Design review of the part built by this model. Coordinates are the model's own, in mm. A direction names the side the tool comes from. Coordinates: 2 decimals unless noted, no trailing zeros. Loops run counter-clockwise (first coordinate to the right, second up) from the corner with the lowest first, then second, coordinate; pieces in that order, holes last. Notation, with made-up numbers: M 78,68.25 L 99,68.25 A18 ccw 99,84.25 Z; hole C 68,86 d2. An arc over 180 degrees is marked long. Answer as a JSON object with one key per item and string values. Group by question number.
1. Consider section C-C (x = 21). State the section outline as (y, z) points, then the cut area to 3 significant figures.
2. Consider section D-D (x = -24). State the section outline as (y, z) points, then the cut area to 3 significant figures.
3. Draft analysis for pull direction Y (two halves, no side actions). For faces 4 (the cylindrical face through (-26.68, 43.93, 5.15)), 5 (the flat face through (-1, 26, 10.16)), 6 (the cylindrical face through (-36.942, 49.272, 4.765)), state which applies: +Y half, -Y half, draft (parallel to the pull), parting line (faces both ways), or undercut.
4. To check wall thickness, follow probe 1 along X at (y, z) = (14, 2); probe 2 along X at (y, z) = (6, 5.5); probe 3 along Z at (x, y) = (-4.5, 31). State the ranges of each line that lie inside material, in increasing order.
5. Machinability: for faces 1 (the flat face through (-21.356, 24, 5)), 2 (the flat face through (-5.56, 16.14, 20.2)), 3 (the flat face through (1.766, 27.835, 21.408)), which of the approach directions +Z, -Z, +X, -X, +Y, -Y give a long, thin tool a straight path to every point of the face, cutting with its end or side? Answer none if there is none.
6. Consider section A-A (x = 29). State the section outline as (y, z) points.
7. Consider section B-B (y = 6.5). State the section outline as (x, z) points.
8. Insertion check: pin 1 (8 mm diameter, centred on x = -30.5, y = 24, fed in from +Z); pin 2 (5 mm diameter, centred on x = -1, y = 37.5, fed in from -Z); pin 3 (3 mm diameter, centred on x = 8.5, z = 20, fed in from -Y); pin 4 (5 mm diameter, centred on y = 39.5, z = 21, fed in from +X). Each pin has a flat end and moves straight along its axis. Give the tip position at first contact, or say it passes through.
from build123d import *

# Parameters (mm, degrees)
F0_W          = 76.2
F0_H          = 50.8
F1_DEPTH      = 10.16
F5_DEPTH      = 23.60986
F5_DEPTH_BACK = 6.00945
F7_DEPTH      = 25.4
F9_D          = 11.43
F9_DEPTH      = 127
F11_D         = 5.08
F11_DEPTH     = 127
F12_R         = 5.08
F13_SIZE      = 0.762
F14_R         = 2.54


with BuildPart() as f1:
    # F0 (on Top) → F1 (new body)
    with BuildSketch(Plane.XY):
        with Locations((-0.290839, 25.4)):
            Rectangle(F0_W, F0_H)
    extrude(amount=F1_DEPTH)

    # F4 (on face) → F5 (join, two sides)
    with BuildSketch(Plane(origin=(-3.34157, 3.876222, 14.060855), x_dir=(0.974746, 0.059349, 0.215288), z_dir=(-0.223318, 0.259049, 0.939693))) as f5_sk:
        Polygon((17.944019, 29.214139), (-2.262714, 12.845073), (2.102678, 7.456231), (22.309411, 23.825297), align=None)
    extrude(amount=F5_DEPTH)
    extrude(f5_sk.sketch, amount=-F5_DEPTH_BACK)

    # F6 (on face) → F7 (cut)
    with BuildSketch(Plane.XY.offset(10.16)):
        with BuildLine():
            ThreePointArc((-21.356091, 38.483839), (-26.801871, 43.92962), (-32.247651, 38.483839))
            Line((-32.247651, 38.483839), (-32.247651, 10.246455))
            ThreePointArc((-32.247651, 10.246455), (-26.801871, 4.800675), (-21.356091, 10.246455))
            Line((-21.356091, 10.246455), (-21.356091, 38.483839))
        make_face()
    extrude(amount=-F7_DEPTH, mode=Mode.SUBTRACT)

    # F9
    with Locations(Plane.XY.offset(10.16)):
        with Locations((28.977718, 9.68211)):
            Hole(F9_D / 2, depth=F9_DEPTH)

    # F11
    with Locations(Plane(origin=(-2.742742, 3.181581, -1.528896), x_dir=(0.789646, 0.553023, -0.265753), z_dir=(0.613563, -0.711733, 0.34202))):
        with Locations((8.980069, 37.900489)):
            Hole(F11_D / 2, depth=F11_DEPTH)

    # F12
    f12_edges = [f1.edges().sort_by_distance(p)[0] for p in [
        (37.809161, 0, 5.08),
        (37.809161, 50.8, 5.08),
        (-38.390839, 50.8, 5.08),
        (-38.390839, 0, 5.08),
    ]]
    fillet(f12_edges, radius=F12_R)

    # F13
    f13_edges = [f1.edges().sort_by_distance(p)[0] for p in [
        (-0.290839, 0, 10.16),
    ]]
    chamfer(f13_edges, length=F13_SIZE)

    # F14
    f14_edges = [f1.edges().sort_by_distance(p)[0] for p in [
        (-8.692086, 19.773218, 33.531991),
        (11.004337, 36.752892, 33.531991),
    ]]
    fillet(f14_edges, radius=F14_R)


solid = f1.part
Findings below:
{
 "1": {"outline": "M 0,0 L 50.8,0 L 50.8,9.4 L 50.04,10.16 L 0.76,10.16 L 0,9.4 Z", "area": "516 mm^2"},
 "2": {"outline": "M 0,0 L 5.58,0 L 5.58,10.16 L 0.76,10.16 L 0,9.4 Z; M 43.15,0 L 50.8,0 L 50.8,9.4 L 50.04,10.16 L 43.15,10.16 Z", "area": "134 mm^2"},
 "3": {"face 4": "undercut", "face 5": "draft", "face 6": "+Y half"},
 "4": {"probe 1": "x = -38.39 to -32.25, -21.36 to 25.23, 32.72 to 37.81", "probe 2": "x = -38.39 to -30.21, -23.39 to 24.61, 33.35 to 37.81", "probe 3": "z = 0 to 10.16"},
 "5": {"face 1": "+Z, -Z", "face 2": "+Z, -X, -Y", "face 3": "-X, +Y"},
 "6": {"outline": "M 0,0 L 3.97,0 L 3.97,10.16 L 0.76,10.16 L 0,9.4 Z; M 15.4,0 L 50.8,0 L 50.8,9.4 L 50.04,10.16 L 15.4,10.16 Z"},
 "7": {"outline": "M -38.39,0 L -30.75,0 L -30.75,10.16 L -37.63,10.16 L -38.39,9.4 Z; M -22.85,0 L 24.23,0 L 24.23,10.16 L -22.85,10.16 Z; M 33.72,0 L 37.81,0 L 37.81,9.4 L 37.05,10.16 L 33.72,10.16 Z"},
 "8": {"pin 1": "stops at z = 10.16", "pin 2": "stops at z = 0", "pin 3": "stops at y = 21.74", "pin 4": "passes through"}
}
